For this review, take the finished solid that the model builds, in its own axes (mm). Round coordinates to 2 decimals unless told otherwise and drop trailing zeros. Order: outer loops, then holes, each group sorted by start corner. A loop starts at its lowest first (then second) coordinate and runs counter-clockwise, first axis right, second up. Notation, with made-up numbers: (79, -4) -> (126, -4) arc R31 cw to (126, 29) -> close; hole circle Ø9 at (-25, -24.5). An arc over 180 degrees is marked (long way). Put each result on its own line as item: value. Start each with the question number.
```python
from build123d import *

# Parameters (mm, degrees)
SKETCH1_W           = 246
SKETCH1_H           = 154
BOSS_EXTRUDE1_DEPTH = 7
SKETCH2_W           = 240
SKETCH2_H           = 148
CUT_EXTRUDE1_DEPTH  = 5
SKETCH3_W           = 220
SKETCH3_H           = 128
CUT_EXTRUDE2_DEPTH  = 5
BOSS_EXTRUDE2_START = -3
SKETCH6_W           = 240
SKETCH6_H           = 68.5
SKETCH6_W_2         = 246
SKETCH6_H_2         = 154
BOSS_EXTRUDE2_DEPTH = 2.5
SKETCH8_W           = 39
SKETCH8_H           = 0.3
SKETCH8_W_2         = 12.26
CUT_EXTRUDE5_DEPTH  = 5
SKETCH9_R           = 0.5
CUT_EXTRUDE6_DEPTH  = 5
SKETCH10_R          = 2.54
CUT_EXTRUDE7_DEPTH  = 5


with BuildPart() as part:
    # Sketch1 → Boss-Extrude1 (new body)
    with BuildSketch(Plane(origin=(0, 0, 0), x_dir=(1, 0, 0), z_dir=(0, 1, 0))):
        Rectangle(SKETCH1_W, SKETCH1_H)
    extrude(amount=-BOSS_EXTRUDE1_DEPTH)

    # Sketch2 → Cut-Extrude1 (cut)
    with BuildSketch(Plane(origin=(0, 0, 0), x_dir=(1, 0, 0), z_dir=(0, 1, 0))):
        Rectangle(SKETCH2_W, SKETCH2_H)
    extrude(amount=-CUT_EXTRUDE1_DEPTH, mode=Mode.SUBTRACT)

    # Sketch3 → Cut-Extrude2 (cut)
    with BuildSketch(Plane(origin=(0, -5, 0), x_dir=(1, 0, 0), z_dir=(0, 1, 0))):
        Rectangle(SKETCH3_W, SKETCH3_H)
    extrude(amount=-CUT_EXTRUDE2_DEPTH, mode=Mode.SUBTRACT)

    # Sketch6 → Boss-Extrude2 (add)
    with BuildSketch(Plane(origin=(0, 0, 0), x_dir=(1, 0, 0), z_dir=(0, 1, 0)).offset(BOSS_EXTRUDE2_START)):
        with BuildLine():
            Line((-128.49, -99.5), (128.49, -99.5))
            ThreePointArc((128.49, -99.5), (140.164332957, -94.664332957), (145, -82.99))
            Line((145, -82.99), (145, 173.99))
            ThreePointArc((145, 173.99), (140.164332957, 185.664332957), (128.49, 190.5))
            Line((128.49, 190.5), (-128.49, 190.5))
            ThreePointArc((-128.49, 190.5), (-140.164332957, 185.664332957), (-145, 173.99))
            Line((-145, 173.99), (-145, -82.99))
            ThreePointArc((-145, -82.99), (-140.164332957, -94.664332957), (-128.49, -99.5))
        make_face()
        with Locations((0, 133.75)):
            Rectangle(SKETCH6_W, SKETCH6_H, mode=Mode.SUBTRACT)
        Rectangle(SKETCH6_W_2, SKETCH6_H_2, mode=Mode.SUBTRACT)
    extrude(amount=-BOSS_EXTRUDE2_DEPTH)

    # Sketch8 → Cut-Extrude5 (cut)
    with BuildSketch(Plane(origin=(0, -5, 0), x_dir=(1, 0, 0), z_dir=(0, 1, 0))):
        with Locations((0.5, -72.95)):
            Rectangle(SKETCH8_W, SKETCH8_H)
        with Locations((-36.13, -72.95)):
            Rectangle(SKETCH8_W_2, SKETCH8_H)
    extrude(amount=-CUT_EXTRUDE5_DEPTH, mode=Mode.SUBTRACT)

    # Sketch9 → Cut-Extrude6 (cut)
    with BuildSketch(Plane(origin=(0, -5, 0), x_dir=(1, 0, 0), z_dir=(0, 1, 0))):
        with Locations(Location((119, -46.2, 0), (0, 0, 270))):
            Circle(SKETCH9_R)
        with Locations(Location((119, -42.7, 0), (0, 0, 270))):
            Circle(SKETCH9_R)
    extrude(amount=-CUT_EXTRUDE6_DEPTH, mode=Mode.SUBTRACT)

    # Sketch10 → Cut-Extrude7 (cut)
    with BuildSketch(Plane(origin=(0, -3, 0), x_dir=(1, 0, 0), z_dir=(0, 1, 0))):
        with Locations(Location((-133.604, 140.242, 0), (0, 0, 270))):
            Circle(SKETCH10_R)
        with Locations(Location((-106.172, 180.12, 0), (0, 0, 270))):
            Circle(SKETCH10_R)
        with Locations(Location((-133.604, -49.242, 0), (0, 0, 90))):
            Circle(SKETCH10_R)
        with Locations(Location((-133.604, 45.5, 0), (0, 0, 270))):
            Circle(SKETCH10_R)
        with Locations(Location((0, 180.12, 0), (0, 0, 270))):
            Circle(SKETCH10_R)
        with Locations(Location((0, -89.12, 0), (0, 0, 90))):
            Circle(SKETCH10_R)
        with Locations(Location((-106.172, -89.12, 0), (0, 0, 90))):
            Circle(SKETCH10_R)
        with Locations(Location((106.172, -89.12, 0), (0, 0, 270))):
            Circle(SKETCH10_R)
        with Locations(Location((133.604, 45.5, 0), (0, 0, 90))):
            Circle(SKETCH10_R)
        with Locations(Location((133.604, -49.242, 0), (0, 0, 270))):
            Circle(SKETCH10_R)
        with Locations(Location((106.172, 180.12, 0), (0, 0, 90))):
            Circle(SKETCH10_R)
        with Locations(Location((133.604, 140.242, 0), (0, 0, 90))):
            Circle(SKETCH10_R)
    extrude(amount=-CUT_EXTRUDE7_DEPTH, mode=Mode.SUBTRACT)


solid = part.part
```
Item 1: Consider section C-C, the plane x = 14.5. Write out the cut boundary in (y, z), plus the area to 3 significant figures.
Item 2: For L1, parallel to Z at x = -10.5, y = -3.5; L2, parallel to X at y = -3.75, z = -4.5; L3, parallel to Z at x = -91, y = -5.75, list the stretches that pass through material, from the lowest coordinate up.
Item 3: Insertion check: pin 1 Ø0.9 at (y, z) = (-2, 23.5) entering from +X; pin 2 Ø0.6 at (x, y) = (-8, -6) entering from +Z; pin 3 Ø8 at (x, z) = (133.604, 49.242) entering from +Y. Each pin has a flat end and moves straight along its axis. Give the tip position at first contact, or say it passes through.
Item 4: Mouldability with a two-part tool opening along X and no side actions: class faces 1 (the face through (-9, -5, 65)), 2 (the face through (140.29, -4.23, -185.54)), 3 (the face through (-1, 0, -75)), 4 (the face through (-140.04, -4.23, -185.79)) as +X half, -X half, draft (parallel to the pull), parting line (faces both ways), or undercut.
Item 5: Consider section B-B, the plane z = -4. Write out the cut boundary in (x, y).
Item 6: Consider section A-A, the plane x = 61.5. Write out the cut boundary in (y, z), plus the area to 3 significant figures.
Evaluation:
1. outline: (-7, -77) -> (-5.5, -77) -> (-5.5, -99.5) -> (-3, -99.5) -> (-3, -77) -> (0, -77) -> (0, -74) -> (-5, -74) -> (-5, -64) -> (-7, -64) -> close; (-7, 64) -> (-5, 64) -> (-5, 72.8) -> (-7, 72.8) -> close; (-7, 73.1) -> (-5, 73.1) -> (-5, 74) -> (0, 74) -> (0, 77) -> (-3, 77) -> (-3, 99.5) -> (-5.5, 99.5) -> (-5.5, 77) -> (-7, 77) -> close; (-5.5, -190.5) -> (-3, -190.5) -> (-3, -168) -> (-5.5, -168) -> close
1. area: 250 mm^2
2. L1: z = -190.5 to -168, -99.5 to -74, 74 to 99.5
2. L2: x = -145 to -120, 120 to 145
2. L3: z = -77 to -64, 64 to 77
3. pin 1: stops at x = 123
3. pin 2: stops at z = 77
3. pin 3: stops at y = -3
4. face 1: undercut
4. face 2: +X half
4. face 3: draft
4. face 4: -X half
5. outline: (-145, -5.5) -> (-123, -5.5) -> (-123, -7) -> (-110, -7) -> (-110, -5) -> (-120, -5) -> (-120, 0) -> (-123, 0) -> (-123, -3) -> (-145, -3) -> close; (110, -7) -> (123, -7) -> (123, -5.5) -> (145, -5.5) -> (145, -3) -> (123, -3) -> (123, 0) -> (120, 0) -> (120, -5) -> (110, -5) -> close
6. outline: (-7, -77) -> (-5.5, -77) -> (-5.5, -99.5) -> (-3, -99.5) -> (-3, -77) -> (0, -77) -> (0, -74) -> (-5, -74) -> (-5, -64) -> (-7, -64) -> close; (-7, 64) -> (-5, 64) -> (-5, 74) -> (0, 74) -> (0, 77) -> (-3, 77) -> (-3, 99.5) -> (-5.5, 99.5) -> (-5.5, 77) -> (-7, 77) -> close; (-5.5, -190.5) -> (-3, -190.5) -> (-3, -168) -> (-5.5, -168) -> close
6. area: 251 mm^2
